from build123d import *

# Parameters (mm, degrees)
SKETCH1_R           = 14.2875
BOSS_EXTRUDE1_DEPTH = 3.175
SKETCH2_W           = 3.175
SKETCH2_H           = 50.8
BOSS_EXTRUDE2_DEPTH = 9.525


with BuildPart() as part:
    # Sketch1 → Boss-Extrude1 (new body)
    with BuildSketch(Plane.XY.offset(309.267180797)):
        with BuildLine():
            Line((51.976784349, -201.484673508), (51.976784349, -150.684673508))
            Line((51.976784349, -150.684673508), (77.376784349, -150.684673508))
            ThreePointArc((77.376784349, -150.684673508), (102.776784349, -176.084673508), (77.376784349, -201.484673508))
            Line((77.376784349, -201.484673508), (51.976784349, -201.484673508))
        make_face()
        with Locations((77.376784349, -176.084673508)):
            Circle(SKETCH1_R, mode=Mode.SUBTRACT)
    extrude(amount=BOSS_EXTRUDE1_DEPTH)

    # Sketch2 → Boss-Extrude2 (add)
    with BuildSketch(Plane.XY.offset(312.442180797)):
        with Locations((53.564284349, -176.084673508)):
            Rectangle(SKETCH2_W, SKETCH2_H)
    extrude(amount=BOSS_EXTRUDE2_DEPTH)


solid = part.part
Read the model definition and answer for the solid it produces. Units are mm, in the model's axes. A direction names the side the tool comes from. Give positions to 0.01 mm unless a question says otherwise; leave off trailing zeros. Write each loop counter-clockwise with the first axis right and the second up, starting at its lowest first coordinate (ties: lowest second). Pieces come first, ordered by that corner, then holes. Notation, with made-up numbers: (19, 12.5) - (48, 12.5) arc R23 cw to (48, 47.5) - close; hole circle Ø9 at (22.5, -11). An arc over 180 degrees is marked (long way). Use CSV: the item, a comma, the result in double quotes. Start each with the question number.
Item 1: Flat-ended cylindrical pins translate along their axes: P1, Ø5, axis at y = -162, z = 316.5, coming from the +X side; P2, Ø4, axis at x = 70, y = -189, coming from the +Z side. Find the tip coordinate at first contact, or state that the pin passes through.
Item 2: For faces 5 (the flat face through (55.152, -176, 317)), 6 (the flat face through (62, -150.685, 312)), determine the directions among +Z, -Z, +X, -X, +Y, -Y from which every point of the face is accessible in a straight line to the end or side of a thin tool.
Item 3: The part is cut by section A-A, the plane x = 64. Give the vertices of the cut face in (y, z).
Item 4: The part is cut by section B-B, the plane y = -168.5. Give the vertices of the cut face in (x, z).
Item 5: The part is cut by section D-D, the plane z = 316.5. Give the vertices of the cut face in (x, y).
Item 6: The mould has two halves that part along Y. Classify faces 1 (the cylindrical face through (102.77, -175.53, 310.83)), 2 (the flat face through (62, -201.485, 312)), 3 (the cylindrical face through (74.28, -190.032, 310.832)), 4 (the flat face through (69, -164, 312.442)): pulls with the +Y half, pulls with the -Y half, needs draft (parallel to the pull), parting line crosses it, or undercut.
Item 7: Consider line 1 (Z direction, x = 56.5, y = -154); line 2 (X direction, y = -181, z = 313.5); line 3 (Y direction, x = 83, z = 312). Determine where each line is inside the solid, lowest interval first.
Item 8: The part is cut by section C-C, the plane x = 73. Give the vertices of the cut face in (y, z).
Taken from the geometry:
1,P1,"x = 55.15"
1,P2,"z = 312.44"
2,face 5,"+Z, +X, +Y, -Y"
2,face 6,"+Z, -Z, +X, -X, +Y"
3,outline,"(-201.48, 309.27) - (-181.1, 309.27) - (-181.1, 312.44) - (-201.48, 312.44) - close; (-171.07, 309.27) - (-150.68, 309.27) - (-150.68, 312.44) - (-171.07, 312.44) - close"
4,outline,"(51.98, 309.27) - (65.27, 309.27) - (65.27, 312.44) - (55.15, 312.44) - (55.15, 321.97) - (51.98, 321.97) - close; (89.48, 309.27) - (101.62, 309.27) - (101.62, 312.44) - (89.48, 312.44) - close"
5,outline,"(51.98, -201.48) - (55.15, -201.48) - (55.15, -150.68) - (51.98, -150.68) - close"
6,face 1,"parting line crosses it"
6,face 2,"pulls with the -Y half"
6,face 3,"undercut"
6,face 4,"needs draft"
7,line 1,"309.27 to 312.44"
7,line 2,"51.98 to 55.15"
7,line 3,"-200.85 to -189.22, -162.95 to -151.31"
8,outline,"(-201.48, 309.27) - (-189.69, 309.27) - (-189.69, 312.44) - (-201.48, 312.44) - close; (-162.48, 309.27) - (-150.68, 309.27) - (-150.68, 312.44) - (-162.48, 312.44) - close"
